The model under review builds one solid part; all positions refer to its coordinate system, in mm. Face numbers are marked on the shaded views. A direction names the side the tool comes from. Round coordinates to 2 decimals unless told otherwise and drop trailing zeros. Write each loop counter-clockwise with the first axis right and the second up, starting at its lowest first coordinate (ties: lowest second). Pieces come first, ordered by that corner, then holes. Notation, with made-up numbers: M -29.5,73 L 18.5,73 A25 cw 18.5,100 Z; hole C 43.5,-9 d7. An arc over 180 degrees is marked long. Write item = value, one per line. Start each with the question number.
Item 1: Take a section at D-D, the plane x = 0. Give the boundary of the cut face in (y, z).
Item 2: Take a section at B-B, the plane y = 30.1. Give the boundary of the cut face in (x, z).
Item 3: Take a section at C-C, the plane z = -4.75. Give the boundary of the cut face in (x, y), plus the area to 3 significant figures.
Item 4: Tool access review of the marked faces 1, 2 and 3: name each direction out of +Z, -Z, +X, -X, +Y, -Y from which nothing blocks a thin tool from reaching the whole face with its end or side.
Item 5: For pin 1 Ø1.5 at (y, z) = (20, 4) entering from +X; pin 2 Ø10 at (x, z) = (5, -15) entering from +Y; pin 3 Ø0.6 at (x, y) = (4.5, 31.5) entering from +Z; pin 4 Ø8 at (x, z) = (-2, -9.5) entering from +Y, all flat-tipped, find the tip position at first contact; note any pin that passes through.
Item 6: Take a section at A-A, the plane z = 29. Give the boundary of the cut face in (x, y), plus the area to 3 significant figures.
Item 7: To check wall thickness, follow line 1 along Z through (x, y) = (0, 1.15); line 2 along Z through (x, y) = (2.5, 4); line 3 along Y through (x, z) = (-4.8, 4.75). State the ranges of each line that lie inside material, in increasing order.
from build123d import *

# Parameters (mm, degrees)
SKETCH1_W            = 45
SKETCH1_H            = 30
BOSS_EXTRUDE1_DEPTH  = 3
SKETCH3_R            = 1.25
BOSS_EXTRUDE2_DEPTH  = 2
SKETCH4_W            = 10.8
SKETCH4_H            = 12
BOSS_EXTRUDE3_DEPTH  = 2
SKETCH10_W           = 18
SKETCH10_H           = 70
BOSS_EXTRUDE4_DEPTH  = 3
SKETCH11_W           = 13.5
SKETCH11_H           = 30
CUT_EXTRUDE1_DEPTH   = 3
M5_CLEARANCE_HOLE1_D = 5.5


with BuildPart() as part:
    # Sketch1 → Boss-Extrude1 (new body)
    with BuildSketch(Plane(origin=(0, 0, 0), x_dir=(1, 0, 0), z_dir=(0, 1, 0))):
        Rectangle(SKETCH1_W, SKETCH1_H)
    extrude(amount=BOSS_EXTRUDE1_DEPTH)

    # Sketch3 → Boss-Extrude2 (add)
    with BuildSketch(Plane(origin=(-3.4, 0, 0), x_dir=(0, 0, -1), z_dir=(1, 0, 0))):
        Polygon((7.5, 40), (-7.5, 40), (-7.5, 15), (-15, 15), (-15, 0), (15, 0), (15, 15), (7.5, 15), align=None)
        with Locations((-4.75, 30.1)):
            Circle(SKETCH3_R, mode=Mode.SUBTRACT)
        with Locations((4.75, 30.1)):
            Circle(SKETCH3_R, mode=Mode.SUBTRACT)
    extrude(amount=-BOSS_EXTRUDE2_DEPTH)

    # Mirror1: part across plane


with BuildPart() as part_1:
    add(part.part)
    add(part.part.mirror(Plane(origin=(0, 0, 0), x_dir=(0, 0, 1), z_dir=(1, 0, 0))))

    # Sketch4 → Boss-Extrude3 (add)
    with BuildSketch(Plane.XY.offset(15)):
        with Locations((0, 9)):
            Rectangle(SKETCH4_W, SKETCH4_H)
    boss_extrude3 = extrude(amount=-BOSS_EXTRUDE3_DEPTH)

    # Mirror2: Boss-Extrude3 across plane
    add(boss_extrude3.mirror(Plane.XY))

    # Sketch10 → Boss-Extrude4 (add)
    with BuildSketch(Plane(origin=(0, 3, 0), x_dir=(1, 0, 0), z_dir=(0, 1, 0))):
        Rectangle(SKETCH10_W, SKETCH10_H)
    extrude(amount=-BOSS_EXTRUDE4_DEPTH)

    # Sketch11 → Cut-Extrude1 (cut)
    with BuildSketch(Plane(origin=(0, 3, 0), x_dir=(1, 0, 0), z_dir=(0, 1, 0))):
        with Locations((-15.75, 0)):
            Rectangle(SKETCH11_W, SKETCH11_H)
    cut_extrude1 = extrude(amount=-CUT_EXTRUDE1_DEPTH, mode=Mode.SUBTRACT)

    # Mirror3: Cut-Extrude1 across plane
    add(cut_extrude1.mirror(Plane(origin=(0, 0, 0), x_dir=(0, 0, 1), z_dir=(1, 0, 0))), mode=Mode.SUBTRACT)

    # M5 Clearance Hole1 (through all)
    with Locations(Plane(origin=(0, 3, 0), x_dir=(1, 0, 0), z_dir=(0, 1, 0))):
        with Locations((0, -29), (0, 29)):
            Hole(M5_CLEARANCE_HOLE1_D / 2)


solid = part_1.part
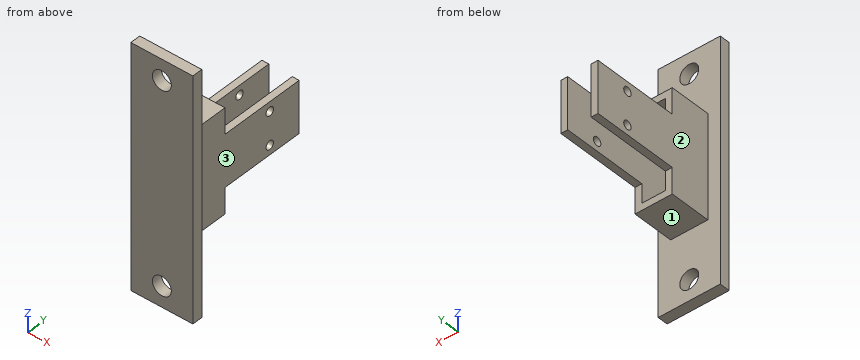
Response values:
q1.outline = M 0,-35 L 3,-35 L 3,-31.75 L 0,-31.75 Z; M 0,-26.25 L 3,-26.25 L 3,-15 L 15,-15 L 15,-13 L 3,-13 L 3,13 L 15,13 L 15,15 L 3,15 L 3,26.25 L 0,26.25 Z; M 0,31.75 L 3,31.75 L 3,35 L 0,35 Z
q2.outline = M -5.4,-7.5 L -3.4,-7.5 L -3.4,-6 L -5.4,-6 Z; M -5.4,-3.5 L -3.4,-3.5 L -3.4,3.5 L -5.4,3.5 Z; M -5.4,6 L -3.4,6 L -3.4,7.5 L -5.4,7.5 Z; M 3.4,-7.5 L 5.4,-7.5 L 5.4,-6 L 3.4,-6 Z; M 3.4,-3.5 L 5.4,-3.5 L 5.4,3.5 L 3.4,3.5 Z; M 3.4,6 L 5.4,6 L 5.4,7.5 L 3.4,7.5 Z
q3.outline = M -9,0 L 9,0 L 9,3 L 5.4,3 L 5.4,28.85 L 3.4,28.85 L 3.4,3 L -3.4,3 L -3.4,28.85 L -5.4,28.85 L -5.4,3 L -9,3 Z; M -5.4,31.35 L -3.4,31.35 L -3.4,40 L -5.4,40 Z; M 3.4,31.35 L 5.4,31.35 L 5.4,40 L 3.4,40 Z
q3.area = 192 mm2
q4.face_1 = -Z, +X, -X, +Y
q4.face_2 = +Z, -Z, -X, +Y
q4.face_3 = +Z, -Z, +X, +Y
q5.pin_1 = 5.4
q5.pin_2 = 15
q5.pin_3 = 7.5
q5.pin_4 = 40
q6.outline = M -9,0 L -2.75,0 L -2.75,3 L -9,3 Z; M 2.75,0 L 9,0 L 9,3 L 2.75,3 Z
q6.area = 37.5 mm2
q7.line_1 = -35 to -31.75, -26.25 to 26.25, 31.75 to 35
q7.line_2 = -15 to -13, 13 to 15
q7.line_3 = 0 to 28.85, 31.35 to 40
